Build history of the part. All positions in model axes, mm. A direction names the side the tool comes from. Coordinates: 2 decimals unless noted, no trailing zeros. Order: outer loops, then holes, each group sorted by start corner. A loop starts at its lowest first (then second) coordinate and runs counter-clockwise, first axis right, second up. Notation, with made-up numbers: (67, 1) - (80, 1) arc R21 ccw to (80, 16) - close; hole circle Ø1 at (-35, -37.75). An arc over 180 degrees is marked (long way). One line per item, written item: value.
from build123d import *

# Parameters (mm, degrees)
F1_DEPTH = 10
F3_DEPTH = 30
F4_W     = 10
F4_H     = 284.7173312026
F5_DEPTH = 30


with BuildPart() as f1:
    # F0 (on Front) → F1 (new body)
    with BuildSketch(Plane.XZ):
        Polygon((-68, 120), (-68, 0), (-15, 0), (-40, 25), (-39.2928932188, 25.7071067812), (-13.5857864376, 0), (56, 0), (56, -69.5857864376), (85.8867522003, -99.4725386379), (85.1796454191, -100.1796454191), (56, -71), (56, -124.05038625), (256, -124.05038625), (109.3597338439, 120), align=None)
        Polygon((-40, 25), (-15, 0), (-13.5857864376, 0), (-39.2928932188, 25.7071067812), align=None)
        Polygon((-13.5857864376, 0), (-15, 0), (56, -71), (56, -69.5857864376), align=None)
        Polygon((56, -69.5857864376), (56, -71), (85.1796454191, -100.1796454191), (85.8867522003, -99.4725386379), align=None)
    extrude(amount=F1_DEPTH)

    # F2 (on face) → F3 (join)
    with BuildSketch(Plane.XZ.offset(10)):
        Polygon((117.9314068509, 125.1503807491), (109.3597338439, 120), (256, -124.05038625), (264.571673007, -118.9000055009), align=None)
    extrude(amount=-F3_DEPTH)

    # F4 (on face) → F5 (join)
    with BuildSketch(Plane(origin=(133.3273650703, 0, 80.1111631094), x_dir=(0, -1, 0), z_dir=(-0.8571673007, 0, -0.5150380749))):
        with Locations((-15, -95.8230163087)):
            Rectangle(F4_W, F4_H)
    extrude(amount=F5_DEPTH)


solid = f1.part
1. Band-saw the part on B-B, the plane x = 22.5. Give the cut face in (y, z).
Values found:
outline: (-10, -37.5) - (0, -37.5) - (0, -36.09) - (-10, -36.09) - close; (-10, 0) - (0, 0) - (0, 120) - (-10, 120) - close
2. 3-axis set-ups, long thin cutter, end or side, ignore diameter. For faces 1 (the face through (-42, -5, 0)), 2 (the face through (155, -5, -124.05)), 3 (the face through (21.694, -4.93, -35.28)), 4 (the face through (171, 10, -11)): which of +Z, -Z, +X, -X, +Y, -Y reach the whole face in a straight line?
Values found:
face 1: -Z, -X, +Y, -Y
face 2: -Z, +X, -X, -Y
face 3: +Y, -Y
face 4: -Z, -X
3. Band-saw the part on A-A, the plane y = -6.5. Give the cut face in (x, z), and give its area (3 significant figures).
Values found:
outline: (-68, 0) - (-15, 0) - (56, -71) - (56, -124.05) - (256, -124.05) - (264.57, -118.9) - (117.93, 125.15) - (109.36, 120) - (-68, 120) - close; hole (-13.59, 0) - (56, -69.59) - (56, 0) - close
area: 48,700 mm2
4. Probe line 1 along Y through (x, z) = (121.5, 43.5); line 2 along Y through (x, z) = (44.5, 33.5); line 3 along Z through (x, y) = (109, -6.5). List the from-to ranges inside material, lowest first.
Values found:
line 1: y = -10 to 0, 10 to 20
line 2: y = -10 to 0
line 3: z = -124.05 to 120
5. Band-saw the part on C-C, the plane z = 24.5. Give the cut face in (x, y), and give its area (3 significant figures).
Values found:
outline: (-68, -10) - (178.41, -10) - (178.41, 20) - (131.74, 20) - (131.74, 10) - (166.74, 10) - (166.74, 0) - (-68, 0) - close
area: 3,050 mm2
6. Flat gauge pins, fed straight in: P1, Ø3, axis at y = -6, z = -37.5, coming from the -X side; P2, Ø10, axis at x = 125, y = 12, coming from the -Z side; P3, Ø8, axis at x = -35.5, y = -6, coming from the -Z side. Where does each tip first touch, or does it go through?
Values found:
P1: stops at x = 21
P2: stops at z = 27.4
P3: stops at z = 0
7. Band-saw the part on D-D, the plane x = 225. Give the cut face in (y, z).
Values found:
outline: (-10, -124.05) - (0, -124.05) - (0, -72.46) - (10, -72.46) - (10, -130.71) - (20, -130.71) - (20, -53.04) - (-10, -53.04) - close
8. Two-plate mould, pull along X, no slides. Class faces 5 (the face through (-68, -5, 61)), 6 (the face through (21, -5, 0)), 7 (the face through (22, -5, 120)): pulls with the +X half, pulls with the -X half, needs draft (parallel to the pull), parting line crosses it, or undercut.
Values found:
face 5: pulls with the -X half
face 6: undercut
face 7: needs draft
